from build123d import *

# Parameters (mm, degrees)
SKETCH_1_W          = 48
SKETCH_1_H          = 20
EXTRUDE_1_DEPTH     = 30
SKETCH_2_W          = 14
SKETCH_2_H          = 30
CUT_EXTRUDE_1_DEPTH = 7
SKETCH_7_W          = 22
SKETCH_7_H          = 30
EXTRUDE_2_DEPTH     = 48
SKETCH_8_W          = 21
SKETCH_8_H          = 30
CUT_EXTRUDE_2_DEPTH = 14
SKETCH_9_W          = 21
SKETCH_9_H          = 30
CUT_EXTRUDE_3_DEPTH = 14
SKETCH_11_W         = 10.2
SKETCH_11_H         = 20.2
CUT_EXTRUDE_4_DEPTH = 56.497747702
SKETCH_13_R         = 4
CUT_EXTRUDE_5_DEPTH = 44.783558558
SKETCH_14_R         = 4
CUT_EXTRUDE_6_DEPTH = 44.783558558
FILLET_1_R          = 7
SKETCH1_W           = 10.2
SKETCH1_H           = 20.2
BOSS_EXTRUDE1_DEPTH = 4
SKETCH_20_R         = 7.5
CUT_EXTRUDE_8_DEPTH = 44.783558558
SKETCH3_R           = 4
CUT_EXTRUDE2_DEPTH  = 57.920997883
CUT_EXTRUDE3_START  = -25
CUT_EXTRUDE3_DEPTH  = 20


with BuildPart() as part:
    # Эскиз1 → Бобышка-Вытянуть1 (new body)
    with BuildSketch(Plane(origin=(0, 0, 0), x_dir=(1, 0, 0), z_dir=(0, 1, 0))):
        Rectangle(SKETCH_1_W, SKETCH_1_H)
    extrude(amount=EXTRUDE_1_DEPTH)

    # Эскиз2 → Вырез-Вытянуть1 (cut)
    with BuildSketch(Plane.XY.offset(10)):
        with Locations((0, 15)):
            Rectangle(SKETCH_2_W, SKETCH_2_H)
    extrude(amount=-CUT_EXTRUDE_1_DEPTH, mode=Mode.SUBTRACT)

    # Эскиз7 → Бобышка-Вытянуть2 (add)
    with BuildSketch(Plane(origin=(24, 0, 0), x_dir=(0, 0, -1), z_dir=(1, 0, 0))):
        with Locations((21, 15)):
            Rectangle(SKETCH_7_W, SKETCH_7_H)
    extrude(amount=-EXTRUDE_2_DEPTH)

    # Эскиз8 → Вырез-Вытянуть2 (cut)
    with BuildSketch(Plane(origin=(24, 0, 0), x_dir=(0, 0, -1), z_dir=(1, 0, 0))):
        with Locations((21.5, 15)):
            Rectangle(SKETCH_8_W, SKETCH_8_H)
    extrude(amount=-CUT_EXTRUDE_2_DEPTH, mode=Mode.SUBTRACT)

    # Эскиз9 → Вырез-Вытянуть3 (cut)
    with BuildSketch(Plane.ZY.offset(24)):
        with Locations((-21.5, 15)):
            Rectangle(SKETCH_9_W, SKETCH_9_H)
    extrude(amount=-CUT_EXTRUDE_3_DEPTH, mode=Mode.SUBTRACT)

    # Эскиз11 → Вырез-Вытянуть4 (cut, through all)
    with BuildSketch(Plane.ZY.offset(10)):
        with Locations((-21.5, 15)):
            Rectangle(SKETCH_11_W, SKETCH_11_H)
    extrude(amount=-CUT_EXTRUDE_4_DEPTH, mode=Mode.SUBTRACT)

    # Эскиз13 → Вырез-Вытянуть5 (cut, through all)
    with BuildSketch(Plane(origin=(0, 0, -11), x_dir=(-1, 0, 0), z_dir=(0, 0, -1))):
        with Locations((17, 15)):
            Circle(SKETCH_13_R)
    extrude(amount=-CUT_EXTRUDE_5_DEPTH, mode=Mode.SUBTRACT)

    # Эскиз14 → Вырез-Вытянуть6 (cut, through all)
    with BuildSketch(Plane(origin=(0, 0, -11), x_dir=(-1, 0, 0), z_dir=(0, 0, -1))):
        with Locations((-17, 15)):
            Circle(SKETCH_14_R)
    extrude(amount=-CUT_EXTRUDE_6_DEPTH, mode=Mode.SUBTRACT)

    # Скругление1
    fillet_1_edges = [part.edges().sort_by_distance(p)[0] for p in [
        (-7, 15, 3),
        (7, 15, 3),
    ]]
    fillet(fillet_1_edges, radius=FILLET_1_R - 0.0001)  # a hair under: the kernel refuses the full size

    # Sketch1 → Boss-Extrude1 (add)
    with BuildSketch(Plane(origin=(10, 0, 0), x_dir=(0, 0, -1), z_dir=(1, 0, 0))):
        with Locations((21.5, 15)):
            Rectangle(SKETCH1_W, SKETCH1_H)
    extrude(amount=-BOSS_EXTRUDE1_DEPTH)

    # Эскиз20 → Вырез-Вытянуть8 (cut, through all)
    with BuildSketch(Plane(origin=(0, 0, -11), x_dir=(-1, 0, 0), z_dir=(0, 0, -1))):
        with Locations((-17, 15)):
            Circle(SKETCH_20_R)
        with Locations((17, 15)):
            Circle(SKETCH_20_R)
    extrude(amount=CUT_EXTRUDE_8_DEPTH, mode=Mode.SUBTRACT)

    # Sketch3 → Cut-Extrude2 (cut, through all)
    with BuildSketch(Plane(origin=(0, 0, -32), x_dir=(-1, 0, 0), z_dir=(0, 0, -1))):
        with Locations(Location((1, 15, 0), (0, 0, 255.522487814))):
            Circle(SKETCH3_R)
    extrude(amount=-CUT_EXTRUDE2_DEPTH, mode=Mode.SUBTRACT)

    # Sketch4 → Cut-Extrude3 (cut)
    with BuildSketch(Plane(origin=(0, 0, -32), x_dir=(-1, 0, 0), z_dir=(0, 0, -1)).offset(CUT_EXTRUDE3_START)):
        Polygon((1, 22.35), (-5.365286718, 18.675), (-5.365286718, 11.325), (1, 7.65), (7.365286718, 11.325), (7.365286718, 18.675), align=None)
    extrude(amount=-CUT_EXTRUDE3_DEPTH, mode=Mode.SUBTRACT)


solid = part.part
Input: part model. Units: mm. Frame: model coordinates. A direction names the side the tool comes from. Round coordinates to 2 decimals unless told otherwise and drop trailing zeros. Order: outer loops, then holes, each group sorted by start corner. A loop starts at its lowest first (then second) coordinate and runs counter-clockwise, first axis right, second up.
1. Mould query, pull axis X, two halves, no side actions, for faces 5 (the face through (2.227, 9.513, -2.225)), 6 (the face through (-10, 25.3, -21.6)), 7 (the face through (24, 15, 0)), 8 (the face through (-1, 11, -29)). Classes: released by +X, released by -X, zero draft, split by the parting line, or undercut.
The answers:
face 5: undercut
face 6: released by -X
face 7: released by +X
face 8: undercut
2. Cut plane D-D, the plane z = 0. Output: boundary loops of the cut face in (x, y) (3 decimals).
The answers:
outline: (-24, 0) - (24, 0) - (24, 30) - (-24, 30) - close; hole circle Ø8 at (-17, 15); hole (-7.365, 11.325) - (-1, 7.65) - (5.365, 11.325) - (5.365, 18.675) - (-1, 22.35) - (-7.365, 18.675) - close; hole circle Ø8 at (17, 15)
3. Cut plane C-C, the plane y = 17. State how many separate pieces and enclosed holes the cut face has, then the cut area to 3 significant figures.
The answers:
separate pieces: 5
enclosed holes: 0
area: 643 mm2
4. Set-up query: faces 1 (the face through (-6, 15, -16.4)), 2 (the face through (-10, 4, -22)), 3 (the face through (-9.5, 15, -29.3)), 4 (the face through (-4.227, 20.487, -0.508)). Return all of +Z, -Z, +X, -X, +Y, -Y with unobstructed straight access to the full face (end or side cutting, diameter ignored); none if empty.
The answers:
face 1: -X
face 2: -Z, -X, +Y, -Y
face 3: -Z, -X
face 4: +Z
5. Material intervals for line 1 (X direction, y = 15, z = -12.5); line 2 (Y direction, x = 17, z = -1.5); line 3 (X direction, y = 14.25, z = -3.5), sorted ascending.
The answers:
line 1: x = -9.5 to -5, 3 to 9.5
line 2: y = 0 to 11, 19 to 30
line 3: x = -24 to -20.93, -13.07 to -7.37, 5.37 to 13.07, 20.93 to 24
6. Pin query (flat end, axial travel): P1, Ø7, axis at x = -16.5, y = 12.5, coming from the -Z side; P2, Ø6.5, axis at x = -0.5, y = 12.5, coming from the +Z side; P3, Ø6, axis at y = 22.5, z = -22, coming from the +X side; P4, Ø13, axis at x = -1, y = 15, coming from the +Z side. Return the tip coordinate at first contact, or that it passes through.
The answers:
P1: stops at z = -11
P2: stops at z = -7
P3: stops at x = 10
P4: stops at z = 10
7. Cut plane B-B, the plane x = -8. Output: boundary loops of the cut face in (y, z), then the cut area to 3 significant figures.
The answers:
outline: (0, -32) - (30, -32) - (30, 10) - (0, 10) - close; hole (4.9, -26.6) - (25.1, -26.6) - (25.1, -16.4) - (4.9, -16.4) - close
area: 1,050 mm2
8. Cut plane A-A, the plane x = -17. Output: boundary loops of the cut face in (y, z).
The answers:
outline: (0, -11) - (11, -11) - (11, 10) - (0, 10) - close; (19, -11) - (30, -11) - (30, 10) - (19, 10) - close
